For this review, use the dimensioned drawing (mm, ordinates from the lowest corner) and the shaded views. Give positions to 0.01 mm unless a question says otherwise; leave off trailing zeros. Order: outer loops, then holes, each group sorted by start corner. A loop starts at its lowest first (then second) coordinate and runs counter-clockwise, first axis right, second up.
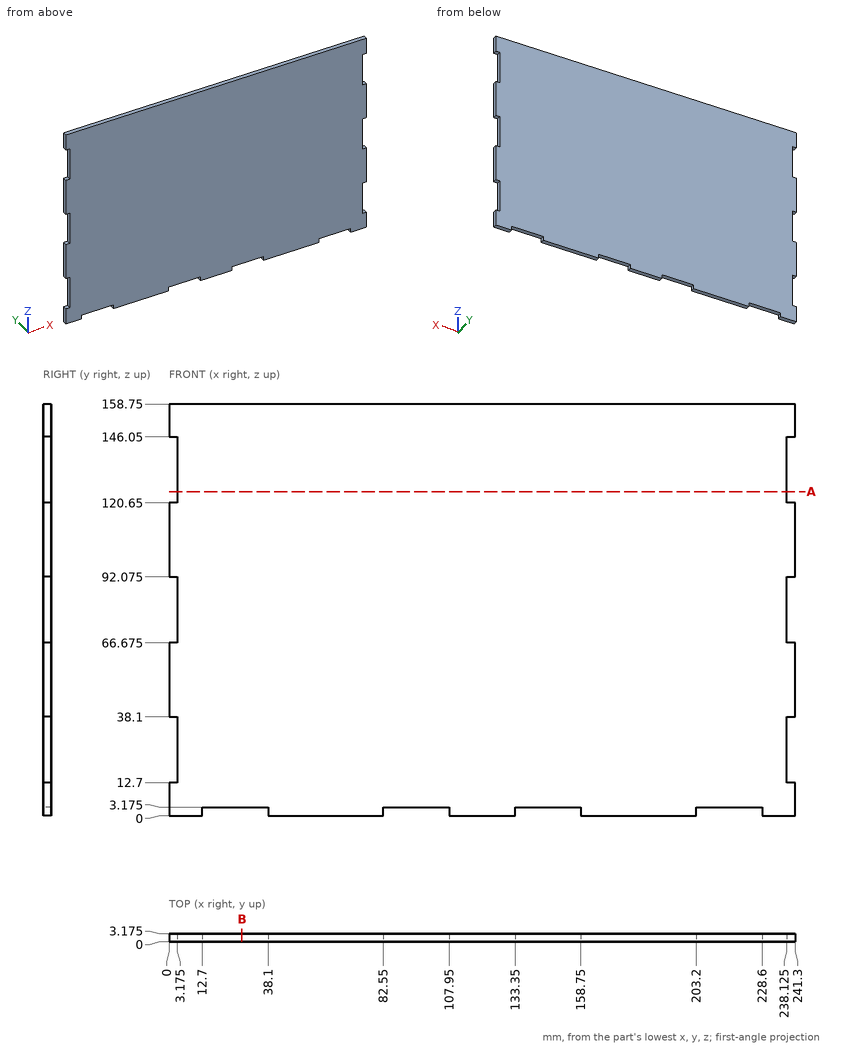
1. Take a section at B-B (x = 28). Write out the cut boundary in (y, z) (3 decimals), and give its area (3 significant figures).
2. Take a section at A-A (z = 125). Write out the cut boundary in (x, y) (3 decimals), and give its area (3 significant figures).
3. Insertion check: pin 1 (1 mm diameter, centred on y = 1, z = 134.5, fed in from +X) (3 decimals); pin 2 (1 mm diameter, centred on x = 86.5, y = 1, fed in from -Z) (3 decimals); pin 3 (1.6 mm diameter, centred on y = 2.5, z = 74, fed in from -X) (3 decimals). Each pin has a flat end and moves straight along its axis. Give the tip position at first contact, or say it passes through.
4. To check wall thickness, follow line 1 (X direction, y = 0.8, z = 143) (3 decimals); line 2 (Z direction, x = 102.5, y = 2.1) (3 decimals). State the ranges of each line that lie inside material, in increasing order.
Answer:
1. outline: (0, 3.175) - (3.175, 3.175) - (3.175, 158.75) - (0, 158.75) - close
1. area: 494 mm2
2. outline: (3.175, 0) - (238.125, 0) - (238.125, 3.175) - (3.175, 3.175) - close
2. area: 746 mm2
3. pin 1: stops at x = 238.125
3. pin 2: stops at z = 3.175
3. pin 3: stops at x = 3.175
4. line 1: x = 3.175 to 238.125
4. line 2: z = 3.175 to 158.75
